Could you check a few things on this model? Use its own coordinates, in mm. Round coordinates to 2 decimals unless told otherwise and drop trailing zeros. Order: outer loops, then holes, each group sorted by start corner. A loop starts at its lowest first (then second) coordinate and runs counter-clockwise, first axis right, second up.
```python
from build123d import *

# Parameters (mm, degrees)
SKETCH1_R                                       = 140
BOSS_EXTRUDE1_DEPTH                             = 12
CSK_FOR_M4_FLAT_HEAD_MACHINE_SCREW1_D           = 4.3
CSK_FOR_M4_FLAT_HEAD_MACHINE_SCREW1_CSINK_D     = 9.4
CSK_FOR_M4_FLAT_HEAD_MACHINE_SCREW1_CSINK_ANGLE = 90


with BuildPart() as part:
    # Sketch1 → Boss-Extrude1 (new body)
    with BuildSketch(Plane.XY):
        Circle(SKETCH1_R)
    extrude(amount=BOSS_EXTRUDE1_DEPTH)

    # CSK for M4 Flat Head Machine Screw1 (through all)
    with Locations(Plane(origin=(0, 0, 0), x_dir=(-1, 0, 0), z_dir=(0, 0, -1))):
        with Locations((0, 135), (135, 0), (0, -135), (-135, 0), (-95.5, 95.5), (95.5, 95.5), (95.5, -95.5), (-95.5, -95.5)):
            CounterSinkHole(CSK_FOR_M4_FLAT_HEAD_MACHINE_SCREW1_D / 2, CSK_FOR_M4_FLAT_HEAD_MACHINE_SCREW1_CSINK_D / 2, counter_sink_angle=CSK_FOR_M4_FLAT_HEAD_MACHINE_SCREW1_CSINK_ANGLE)


solid = part.part
```
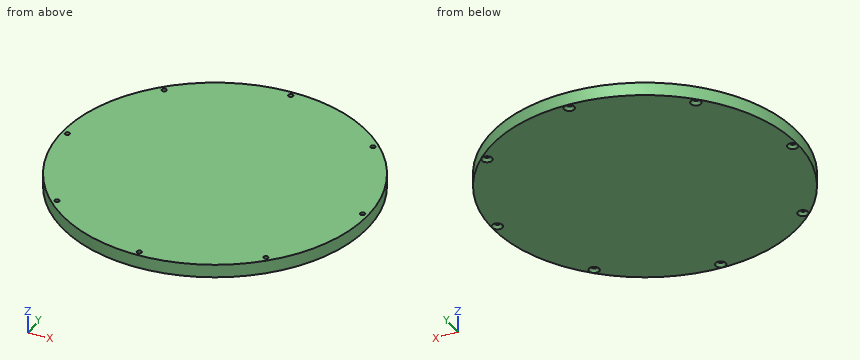
Q1. I need wall thicknesses on L1, parallel to Y at x = 0, z = 7; L2, parallel to X at y = 95.5, z = 4.75. Which ranges of each line are inside material? Lowest first, please.
Q2. Imagine slicing it at B-B, the plane x = -45.5. Please give me the cut outline in (y, z), then the cut area to 3 significant figures.
Q3. Imagine slicing it at C-C, the plane y = -86.5. Please give me the cut outline in (x, z), then the cut area to 3 significant figures.
Q4. Imagine slicing it at A-A, the plane z = 5.25. State how many separate pieces and enclosed holes the cut face has, then the cut area to 3 significant figures.
Q5. For P1, Ø4, axis at x = 56, z = 1.5, coming from the +Y side; P2, Ø5, axis at x = 0, y = -135, coming from the -Z side; P3, Ø2, axis at y = -56, z = 9.5, coming from the +X side, each with a flat end and sliding along its axis, tell me the tip position at first contact or that it passes through.
Filled in:
1. L1: y = -140 to -137.15, -132.85 to 132.85, 137.15 to 140
1. L2: x = -102.37 to -97.65, -93.35 to 93.35, 97.65 to 102.37
2. outline: (-132.4, 0) - (132.4, 0) - (132.4, 12) - (-132.4, 12) - close
2. area: 3,180 mm2
3. outline: (-110.08, 0) - (110.08, 0) - (110.08, 12) - (-110.08, 12) - close
3. area: 2,640 mm2
4. separate pieces: 1
4. enclosed holes: 8
4. area: 61,500 mm2
5. P1: stops at y = 129.17
5. P2: stops at z = 2.2
5. P3: stops at x = 128.74
